from build123d import *

# Parameters (mm, degrees)
F0_W     = 60
F0_H     = 12
F1_DEPTH = 40
F0_R     = 7.5
F2_DEPTH = 10
F3_R     = 5
F4_DEPTH = 12


with BuildPart() as f1:
    # F0 (on Front) → F1 (new body)
    with BuildSketch(Plane.XZ):
        with Locations((30, 6)):
            Rectangle(F0_W, F0_H)
    extrude(amount=F1_DEPTH)

    # F0 (on Front) → F2 (join)
    with BuildSketch(Plane.XZ):
        with BuildLine():
            Line((36, 39), (0, 12))
            Line((0, 12), (60, 12))
            Line((60, 12), (60, 27))
            ThreePointArc((60, 27), (51.708204, 40.416408), (36, 39))
        make_face()
        with Locations((45, 27)):
            Circle(F0_R, mode=Mode.SUBTRACT)
    extrude(amount=F2_DEPTH)

    # F3 (on face) → F4 (cut, through all)
    with BuildSketch(Plane.XY.offset(12)):
        with Locations((15, -25)):
            Circle(F3_R)
        with Locations((45, -25)):
            Circle(F3_R)
    extrude(amount=-F4_DEPTH, mode=Mode.SUBTRACT)


solid = f1.part
Source: CAD feature listing. Evaluate the final solid. Frame: model axes, mm. A direction names the side the tool comes from. Round coordinates to 2 decimals unless told otherwise and drop trailing zeros. Order: outer loops, then holes, each group sorted by start corner. A loop starts at its lowest first (then second) coordinate and runs counter-clockwise, first axis right, second up. Notation, with made-up numbers: (32.25, -14.75) - (47.25, -14.75) arc R11 ccw to (47.25, -4.75) - close; hole circle Ø11 at (70, 64.5). An arc over 180 degrees is marked (long way). Use a Markdown table: item, result. Add a question column.
1. Line query: probe 1 along Z at (x, y) = (45, -6); probe 2 along Y at (x, z) = (15, 9.25); probe 3 along Y at (x, z) = (26.5, 29). Output: solid intervals per line, ascending.
2. Section query D-D (z = 28.5). Return the cut outline in (x, y), then the cut area to 3 significant figures.
3. Set-up query: faces 5 (the cylindrical face through (17.307, -29.436, 6.084)), 6 (the flat face through (30, -25, 12)). Return all of +Z, -Z, +X, -X, +Y, -Y with unobstructed straight access to the full face (end or side cutting, diameter ignored); none if empty.
4. First-contact query: pin 1 (16 mm diameter, centred on x = 45, y = -25, fed in from +Z); pin 2 (9 mm diameter, centred on x = 20.5, z = 24, fed in from -Y); pin 3 (8 mm diameter, centred on x = 8, y = -6.5, fed in from +Z); pin 4 (9 mm diameter, centred on x = 15, y = -25, fed in from -Z). Flat tips, straight axial feed; report the tip coordinate or a pass-through.
5. Section query C-C (y = -25). Return the cut outline in (x, z).
6. Mould query, pull axis X, two halves, no side actions, for faces 1 (the flat face through (60, -15, 7)), 2 (the cylindrical face through (52.154, -4.93, 29.253)), 3 (the flat face through (18.252, -4.93, 25.689)), 4 (the flat face through (36, 0, 17)). Classes: +X half, -X half, draft (parallel to the pull), parting line (faces both ways), or undercut.
7. Section query A-A (x = 45). Return the cut outline in (y, z), then the cut area to 3 significant figures.
8. Section query B-B (x = 15). Return the cut outline in (y, z).
Derived:
| question | item | result |
|---|---|---|
| 1 | probe 1 | 0 to 19.5, 34.5 to 42 |
| 1 | probe 2 | -40 to -30, -20 to 0 |
| 1 | probe 3 | -10 to 0 |
| 2 | outline | (22, -10) - (37.65, -10) - (37.65, 0) - (22, 0) - close; (52.35, -10) - (59.92, -10) - (59.92, 0) - (52.35, 0) - close |
| 2 | area | 232 mm2 |
| 3 | face 5 | +Z, -Z |
| 3 | face 6 | +Z, +X, -X, -Y |
| 4 | pin 1 | z = 12 |
| 4 | pin 2 | y = -10 |
| 4 | pin 3 | z = 21 |
| 4 | pin 4 | through |
| 5 | outline | (0, 0) - (10, 0) - (10, 12) - (0, 12) - close; (20, 0) - (40, 0) - (40, 12) - (20, 12) - close; (50, 0) - (60, 0) - (60, 12) - (50, 12) - close |
| 6 | face 1 | +X half |
| 6 | face 2 | undercut |
| 6 | face 3 | -X half |
| 6 | face 4 | draft |
| 7 | outline | (-40, 0) - (-30, 0) - (-30, 12) - (-40, 12) - close; (-20, 0) - (0, 0) - (0, 19.5) - (-10, 19.5) - (-10, 12) - (-20, 12) - close; (-10, 34.5) - (0, 34.5) - (0, 42) - (-10, 42) - close |
| 7 | area | 510 mm2 |
| 8 | outline | (-40, 0) - (-30, 0) - (-30, 12) - (-40, 12) - close; (-20, 0) - (0, 0) - (0, 23.25) - (-10, 23.25) - (-10, 12) - (-20, 12) - close |
